Read the model definition and answer for the solid it produces. Units are mm, in the model's axes. Face numbers are marked on the shaded views. Give positions to 0.01 mm unless a question says otherwise; leave off trailing zeros. Order: outer loops, then holes, each group sorted by start corner. A loop starts at its lowest first (then second) coordinate and runs counter-clockwise, first axis right, second up.
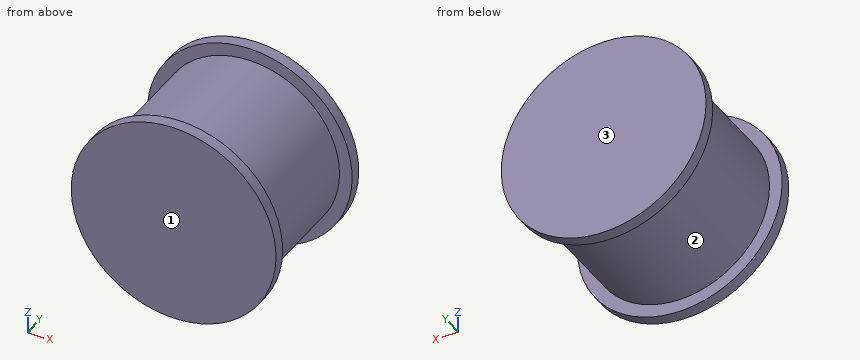
```python
from build123d import *

# Parameters (mm, degrees)
SKETCH_1_R      = 15.35
EXTRUDE_1_DEPTH = 10.5
SKETCH_2_R      = 17.5
EXTRUDE_2_DEPTH = 2


with BuildPart() as part:
    # 草图1 → 凸台-拉伸1 (new, symmetric)
    with BuildSketch(Plane(origin=(0, 0, 0), x_dir=(1, 0, 0), z_dir=(0, 1, 0))):
        with Locations(Location((0, 0, 0), (0, 0, 90))):
            Circle(SKETCH_1_R)
    extrude(amount=EXTRUDE_1_DEPTH, both=True)

    # 草图2 → 凸台-拉伸2 (add)
    with BuildSketch(Plane(origin=(0, 10.5, 0), x_dir=(1, 0, 0), z_dir=(0, 1, 0))):
        with Locations(Location((0, 0, 0), (0, 0, 270))):
            Circle(SKETCH_2_R)
    extrude_2 = extrude(amount=EXTRUDE_2_DEPTH)

    # 镜向1: 凸台-拉伸2 across plane
    add(extrude_2.mirror(Plane.ZX))


solid = part.part
```
1) The part is cut by section B-B on x = 0. Determine the outline of the cut face in (y, z).
Final values:
outline: (-12.5, -17.5) - (-10.5, -17.5) - (-10.5, -15.35) - (10.5, -15.35) - (10.5, -17.5) - (12.5, -17.5) - (12.5, 17.5) - (10.5, 17.5) - (10.5, 15.35) - (-10.5, 15.35) - (-10.5, 17.5) - (-12.5, 17.5) - close
2) Given pin 1 (5 mm diameter, centred on x = -5, y = 2.5, fed in from -Z); pin 2 (3 mm diameter, centred on x = -7, y = 7.5, fed in from +Z); pin 3 (10 mm diameter, centred on x = -10.5, y = 7, fed in from -Z), each flat-ended and moving along its own axis, determine where each tip first touches the part or whether it passes through.
Final values:
pin 1: stops at z = -15.15
pin 2: stops at z = 14.33
pin 3: stops at z = -16.07
3) The part is cut by section A-A on z = 0. Determine the outline of the cut face in (x, y), and give its area (3 significant figures).
Final values:
outline: (-17.5, -12.5) - (17.5, -12.5) - (17.5, -10.5) - (15.35, -10.5) - (15.35, 10.5) - (17.5, 10.5) - (17.5, 12.5) - (-17.5, 12.5) - (-17.5, 10.5) - (-15.35, 10.5) - (-15.35, -10.5) - (-17.5, -10.5) - close
area: 785 mm2
4) Consider L1, parallel to Y at x = -13.5, z = 11; L2, parallel to Z at x = 12, y = -4.25; L3, parallel to X at y = 10.25, z = 5. Determine where each line is inside the solid, lowest interval first.
Final values:
L1: y = -12.5 to -10.5, 10.5 to 12.5
L2: z = -9.57 to 9.57
L3: x = -14.51 to 14.51
5) The part is cut by section C-C on y = 8.5. Determine the outline of the cut face in (x, z), and give its area (3 significant figures).
Final values:
outline: circle Ø30.7 at (0, 0)
area: 740 mm2
6) For a pull along Y with two mould halves and no side action, classify the marked faces 1, 2 and 3 as released by +Y, released by -Y, zero draft, split by the parting line, or undercut.
Final values:
face 1: released by -Y
face 2: undercut
face 3: released by +Y
